Model file for the job. Use its own axes, mm. Face numbers are marked on the shaded views. A direction names the side the tool comes from. Round coordinates to 2 decimals unless told otherwise and drop trailing zeros. Order: outer loops, then holes, each group sorted by start corner. A loop starts at its lowest first (then second) coordinate and runs counter-clockwise, first axis right, second up. Notation, with made-up numbers: (-27.5, 62.5) -> (26.5, 62.5) arc R26 cw to (26.5, 89.5) -> close; hole circle Ø7 at (46.25, 3.25). An arc over 180 degrees is marked (long way). Put each result on its own line as item: value. Start each with the question number.
Q1. Cut at B-B, the plane z = 6. List the corners of the cut face in (x, y) (3 decimals), and give its area (3 significant figures).
Q2. Cut at C-C, the plane y = 27. List the corners of the cut face in (x, z), and give its area (3 significant figures).
Q3. Flat gauge pins, fed straight in: P1, Ø6, axis at y = 14, z = -15, coming from the +X side; P2, Ø6, axis at x = 5, y = 40.5, coming from the +Z side; P3, Ø12, axis at x = 13.5, y = 26, coming from the -Z side. Where does each tip first touch, or does it go through?
Q4. Cut at A-A, the plane x = 3. List the corners of the cut face in (y, z) (3 decimals), and give its area (3 significant figures).
Q5. 3-axis set-ups, long thin cutter, end or side, ignore diameter. For the marked faces 1, 2, 3 and 4: which of +Z, -Z, +X, -X, +Y, -Y reach the whole face in a straight line?
Q6. Cut at D-D, the plane z = -10.5. List the corners of the cut face in (x, y) (3 decimals), and give its area (3 significant figures).
Q7. Probe L1, parallel to Z at x = 16.5, y = 39.5; L2, parallel to Z at x = 11, y = 36; L3, parallel to X at y = 10, z = -10. List the from-to ranges inside material, lowest first.
from build123d import *

# Parameters (mm, degrees)
SKETCH1_R           = 19.05
BOSS_EXTRUDE1_DEPTH = 47.625
CUT_EXTRUDE1_DEPTH  = 55.716959208


with BuildPart() as part:
    # Sketch1 → Boss-Extrude1 (new body)
    with BuildSketch(Plane(origin=(0, 0, 0), x_dir=(1, 0, 0), z_dir=(0, 1, 0))):
        with Locations(Location((0, 0, 0), (0, 0, 270))):
            Circle(SKETCH1_R)
    extrude(amount=BOSS_EXTRUDE1_DEPTH)

    # Sketch2 → Cut-Extrude1 (cut, through all)
    with BuildSketch(Plane.XY):
        with BuildLine():
            Line((-19.05, -1.366), (19.05, -1.366))
            Line((19.05, -1.366), (19.05, 29.21))
            ThreePointArc((19.05, 29.21), (12.314807909, 26.420192091), (9.525, 19.685))
            Line((9.525, 19.685), (9.525, 9.525))
            ThreePointArc((9.525, 9.525), (0, 0), (-9.525, 9.525))
            Line((-9.525, 9.525), (-9.525, 19.685))
            ThreePointArc((-9.525, 19.685), (-12.314807909, 26.420192091), (-19.05, 29.21))
            Line((-19.05, 29.21), (-19.05, -1.366))
        make_face()
    extrude(amount=CUT_EXTRUDE1_DEPTH, mode=Mode.SUBTRACT)


solid = part.part
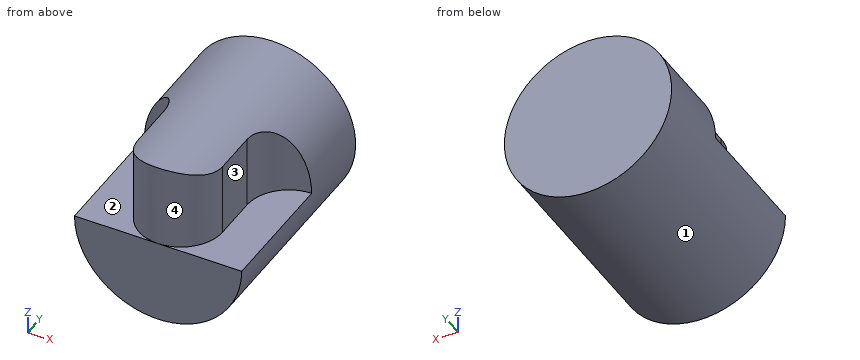
Ans:
1. outline: (-18.08, 29.161) arc R9.525 cw to (-9.525, 19.685) -> (-9.525, 9.525) arc R9.525 ccw to (9.525, 9.525) -> (9.525, 19.685) arc R9.525 cw to (18.08, 29.161) -> (18.08, 47.625) -> (-18.08, 47.625) -> close
1. area: 1,220 mm^2
2. outline: (-19.05, 0) arc R19.05 ccw to (19.05, 0) -> (12.95, 0) -> (12.95, 13.97) arc R19.05 ccw to (-12.95, 13.97) -> (-12.95, 0) -> close
2. area: 1,020 mm^2
3. P1: stops at x = 14.8
3. P2: stops at z = 18.94
3. P3: stops at z = -17.51
4. outline: (0, -18.812) -> (47.625, -18.812) -> (47.625, 18.812) -> (0.485, 18.812) -> (0.485, 0) -> (0, 0) -> close
4. area: 1,780 mm^2
5. face 1: +Y, -Y
5. face 2: +Z, -X, -Y
5. face 3: +Z, +X, -Y
5. face 4: +Z, -Y
6. outline: (-15.895, 0) -> (15.895, 0) -> (15.895, 47.625) -> (-15.895, 47.625) -> close
6. area: 1,510 mm^2
7. L1: z = -9.52 to 9.52
7. L2: z = -15.55 to 15.55
7. L3: x = -16.21 to 16.21
